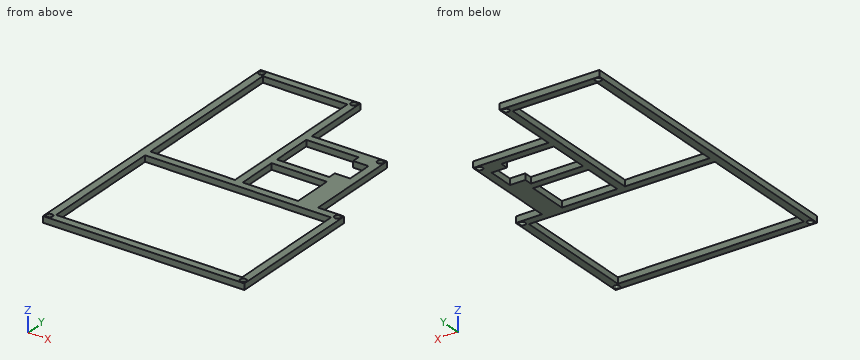
from build123d import *

# Parameters (mm, degrees)
F0_W     = 5
F0_H     = 5
F1_DEPTH = 4


with BuildPart() as f1:
    # F0 (on Top) → F1 (new body)
    with BuildSketch(Plane.XY):
        with BuildLine():
            Line((82.7990943193, -150.3260023594), (82.7990943193, -150.8260023594))
            Line((82.7990943193, -150.8260023594), (85.2990943193, -150.8260023594))
            Line((85.2990943193, -150.8260023594), (85.2990943193, -148.3260023594))
            Line((85.2990943193, -148.3260023594), (84.7990943193, -148.3260023594))
            ThreePointArc((84.7990943193, -148.3260023594), (84.2133078817, -149.7402159218), (82.7990943193, -150.3260023594))
        make_face()
        with BuildLine():
            Line((-45.2009056807, -148.3260023594), (-45.7009056807, -148.3260023594))
            Line((-45.7009056807, -148.3260023594), (-45.7009056807, -150.8260023594))
            Line((-45.7009056807, -150.8260023594), (-43.2009056807, -150.8260023594))
            Line((-43.2009056807, -150.8260023594), (-43.2009056807, -150.3260023594))
            ThreePointArc((-43.2009056807, -150.3260023594), (-44.615119243, -149.7402159218), (-45.2009056807, -148.3260023594))
        make_face()
        with BuildLine():
            Line((-43.2009056807, 49.1739976406), (-43.2009056807, 49.6739976406))
            Line((-43.2009056807, 49.6739976406), (-45.7009056807, 49.6739976406))
            Line((-45.7009056807, 49.6739976406), (-45.7009056807, 47.1739976406))
            Line((-45.7009056807, 47.1739976406), (-45.2009056807, 47.1739976406))
            ThreePointArc((-45.2009056807, 47.1739976406), (-44.615119243, 48.588211203), (-43.2009056807, 49.1739976406))
        make_face()
        with BuildLine():
            Line((85.2990943193, -61.3260023594), (85.2990943193, -58.8260023594))
            Line((85.2990943193, -58.8260023594), (82.7990943193, -58.8260023594))
            Line((82.7990943193, -58.8260023594), (82.7990943193, -59.3260023594))
            ThreePointArc((82.7990943193, -59.3260023594), (84.2133078817, -59.911788797), (84.7990943193, -61.3260023594))
            Line((84.7990943193, -61.3260023594), (85.2990943193, -61.3260023594))
        make_face()
        with BuildLine():
            Line((19.2990943193, 49.6739976406), (16.7990943193, 49.6739976406))
            Line((16.7990943193, 49.6739976406), (16.7990943193, 49.1739976406))
            ThreePointArc((16.7990943193, 49.1739976406), (18.2133078817, 48.588211203), (18.7990943193, 47.1739976406))
            Line((18.7990943193, 47.1739976406), (19.2990943193, 47.1739976406))
            Line((19.2990943193, 47.1739976406), (19.2990943193, 49.6739976406))
        make_face()
        with BuildLine():
            Line((85.2990943193, -63.8260023594), (85.2990943193, -61.3260023594))
            Line((85.2990943193, -61.3260023594), (84.7990943193, -61.3260023594))
            ThreePointArc((84.7990943193, -61.3260023594), (81.384880757, -62.7402159218), (82.7990943193, -59.3260023594))
            Line((82.7990943193, -59.3260023594), (82.7990943193, -58.8260023594))
            Line((82.7990943193, -58.8260023594), (80.2990943193, -58.8260023594))
            Line((80.2990943193, -58.8260023594), (80.2990943193, -63.8260023594))
            Line((80.2990943193, -63.8260023594), (85.2990943193, -63.8260023594))
        make_face()
        with BuildLine():
            Line((14.2990943193, 49.6739976406), (14.2990943193, 44.6739976406))
            Line((14.2990943193, 44.6739976406), (16.7990943193, 44.6739976406))
            Line((16.7990943193, 44.6739976406), (19.2990943193, 44.6739976406))
            Line((19.2990943193, 44.6739976406), (19.2990943193, 47.1739976406))
            Line((19.2990943193, 47.1739976406), (18.7990943193, 47.1739976406))
            ThreePointArc((18.7990943193, 47.1739976406), (15.384880757, 45.7597840782), (16.7990943193, 49.1739976406))
            Line((16.7990943193, 49.1739976406), (16.7990943193, 49.6739976406))
            Line((16.7990943193, 49.6739976406), (14.2990943193, 49.6739976406))
        make_face()
        with BuildLine():
            Line((-37.7009056807, -58.8260023594), (-40.7009056807, -58.8260023594))
            Line((-40.7009056807, -58.8260023594), (-40.7009056807, -52.8260023594))
            Line((-40.7009056807, -52.8260023594), (-40.7009056807, 28.4739976406))
            Line((-40.7009056807, 28.4739976406), (-40.7009056807, 44.6739976406))
            Line((-40.7009056807, 44.6739976406), (14.2990943193, 44.6739976406))
            Line((14.2990943193, 44.6739976406), (14.2990943193, 49.6739976406))
            Line((14.2990943193, 49.6739976406), (-43.2009056807, 49.6739976406))
            Line((-43.2009056807, 49.6739976406), (-43.2009056807, 49.1739976406))
            ThreePointArc((-43.2009056807, 49.1739976406), (-41.7866921183, 48.588211203), (-41.2009056807, 47.1739976406))
            ThreePointArc((-41.2009056807, 47.1739976406), (-43.2009056807, 45.1739976406), (-45.2009056807, 47.1739976406))
            Line((-45.2009056807, 47.1739976406), (-45.7009056807, 47.1739976406))
            Line((-45.7009056807, 47.1739976406), (-45.7009056807, -148.3260023594))
            Line((-45.7009056807, -148.3260023594), (-45.2009056807, -148.3260023594))
            ThreePointArc((-45.2009056807, -148.3260023594), (-43.2009056807, -146.3260023594), (-41.2009056807, -148.3260023594))
            ThreePointArc((-41.2009056807, -148.3260023594), (-41.7866921183, -149.7402159218), (-43.2009056807, -150.3260023594))
            Line((-43.2009056807, -150.3260023594), (-43.2009056807, -150.8260023594))
            Line((-43.2009056807, -150.8260023594), (82.7990943193, -150.8260023594))
            Line((82.7990943193, -150.8260023594), (82.7990943193, -150.3260023594))
            ThreePointArc((82.7990943193, -150.3260023594), (81.384880757, -146.911788797), (84.7990943193, -148.3260023594))
            Line((84.7990943193, -148.3260023594), (85.2990943193, -148.3260023594))
            Line((85.2990943193, -148.3260023594), (85.2990943193, -63.8260023594))
            Line((85.2990943193, -63.8260023594), (80.2990943193, -63.8260023594))
            Line((80.2990943193, -63.8260023594), (80.2990943193, -58.8260023594))
            Line((80.2990943193, -58.8260023594), (68.2990943193, -58.8260023594))
            Line((68.2990943193, -58.8260023594), (68.2990943193, -22.3260023594))
            Line((68.2990943193, -22.3260023594), (68.2990943193, -5.3260023594))
            Line((68.2990943193, -5.3260023594), (63.2990943193, -5.3260023594))
            Line((63.2990943193, -5.3260023594), (63.2990943193, -22.3260023594))
            Line((63.2990943193, -22.3260023594), (53.2990943193, -22.3260023594))
            Line((53.2990943193, -22.3260023594), (53.2990943193, -25.3760023594))
            Line((53.2990943193, -25.3760023594), (53.2990943193, -27.3260023594))
            Line((53.2990943193, -27.3260023594), (51.3490943193, -27.3260023594))
            Line((51.3490943193, -27.3260023594), (28.5490943193, -27.3260023594))
            Line((28.5490943193, -27.3260023594), (19.2990943193, -27.3260023594))
            Line((19.2990943193, -27.3260023594), (19.2990943193, -25.3760023594))
            Line((19.2990943193, -25.3760023594), (19.2990943193, -2.2760023594))
            Line((19.2990943193, -2.2760023594), (19.2990943193, -0.3260023594))
            Line((19.2990943193, -0.3260023594), (14.2990943193, -0.3260023594))
            Line((14.2990943193, -0.3260023594), (14.2990943193, -27.3260023594))
            Line((14.2990943193, -27.3260023594), (14.2990943193, -32.3260023594))
            Line((14.2990943193, -32.3260023594), (14.2990943193, -47.2260023594))
            Line((14.2990943193, -47.2260023594), (14.2990943193, -58.8260023594))
            Line((14.2990943193, -58.8260023594), (11.2990943193, -58.8260023594))
            Line((11.2990943193, -58.8260023594), (-37.7009056807, -58.8260023594))
        make_face()
        Polygon((76.8990943193, -63.8260023594), (80.2990943193, -63.8260023594), (80.2990943193, -67.2260023594), (80.2990943193, -142.4260023594), (80.2990943193, -145.8260023594), (76.8990943193, -145.8260023594), (-37.3009056807, -145.8260023594), (-40.7009056807, -145.8260023594), (-40.7009056807, -142.4260023594), (-40.7009056807, -67.2260023594), (-40.7009056807, -63.8260023594), (-37.3009056807, -63.8260023594), (14.2990943193, -63.8260023594), (19.2990943193, -63.8260023594), align=None, mode=Mode.SUBTRACT)
        Polygon((53.5990943193, -58.8260023594), (19.2990943193, -58.8260023594), (19.2990943193, -32.3260023594), (53.5990943193, -32.3260023594), (55.2990943193, -32.3260023594), (55.2990943193, -34.0260023594), (55.2990943193, -57.1260023594), (55.2990943193, -58.8260023594), align=None, mode=Mode.SUBTRACT)
        with Locations((16.7990943193, 2.1739976406)):
            Rectangle(F0_W, F0_H)
        Polygon((16.7990943193, 44.6739976406), (14.2990943193, 44.6739976406), (14.2990943193, 29.8739976406), (14.2990943193, 4.6739976406), (19.2990943193, 4.6739976406), (19.2990943193, 44.6739976406), align=None)
        with BuildLine():
            Line((65.7990943193, 4.6739976406), (19.2990943193, 4.6739976406))
            Line((19.2990943193, 4.6739976406), (19.2990943193, -0.3260023594))
            Line((19.2990943193, -0.3260023594), (28.5490943193, -0.3260023594))
            Line((28.5490943193, -0.3260023594), (51.3490943193, -0.3260023594))
            Line((51.3490943193, -0.3260023594), (53.2990943193, -0.3260023594))
            Line((53.2990943193, -0.3260023594), (53.2990943193, -2.2760023594))
            Line((53.2990943193, -2.2760023594), (53.2990943193, -5.3260023594))
            Line((53.2990943193, -5.3260023594), (63.2990943193, -5.3260023594))
            Line((63.2990943193, -5.3260023594), (68.2990943193, -5.3260023594))
            Line((68.2990943193, -5.3260023594), (68.2990943193, 2.1739976406))
            Line((68.2990943193, 2.1739976406), (67.7990943193, 2.1739976406))
            ThreePointArc((67.7990943193, 2.1739976406), (64.384880757, 0.7597840782), (65.7990943193, 4.1739976406))
            Line((65.7990943193, 4.1739976406), (65.7990943193, 4.6739976406))
        make_face()
        with BuildLine():
            Line((68.2990943193, 4.6739976406), (65.7990943193, 4.6739976406))
            Line((65.7990943193, 4.6739976406), (65.7990943193, 4.1739976406))
            ThreePointArc((65.7990943193, 4.1739976406), (67.2133078817, 3.588211203), (67.7990943193, 2.1739976406))
            Line((67.7990943193, 2.1739976406), (68.2990943193, 2.1739976406))
            Line((68.2990943193, 2.1739976406), (68.2990943193, 4.6739976406))
        make_face()
    extrude(amount=F1_DEPTH)


solid = f1.part
Geometry check sheet. Reference: the model listing, model coordinates, mm. Give positions to 0.01 mm unless a question says otherwise; leave off trailing zeros. Write each loop counter-clockwise with the first axis right and the second up, starting at its lowest first coordinate (ties: lowest second). Pieces come first, ordered by that corner, then holes.
1) Go/stop test with flat-tipped pins: pin 1 Ø2 at (x, z) = (38.5, 1) entering from +Y; pin 2 Ø1.2 at (y, z) = (17, 1.5) entering from +X; pin 3 Ø2 at (y, z) = (-48.5, 2) entering from +X; pin 4 Ø5 at (x, y) = (55.5, -21.5) entering from +Z. Record where each tip stops, or that it passes through.
Values follow:
pin 1: stops at y = 4.67
pin 2: stops at x = 19.3
pin 3: stops at x = 68.3
pin 4: stops at z = 4
2) Cross-section at C-C (x = -6). Record the boundary of the cut face in (y, z), plus the area to 3 significant figures.
Values follow:
outline: (-150.83, 0) - (-145.83, 0) - (-145.83, 4) - (-150.83, 4) - close; (-63.83, 0) - (-58.83, 0) - (-58.83, 4) - (-63.83, 4) - close; (44.67, 0) - (49.67, 0) - (49.67, 4) - (44.67, 4) - close
area: 60.0 mm2
3) Cross-section at B-B (y = -34.5). Record the boundary of the cut face in (x, z), plus the area to 3 significant figures.
Values follow:
outline: (-45.7, 0) - (-40.7, 0) - (-40.7, 4) - (-45.7, 4) - close; (14.3, 0) - (19.3, 0) - (19.3, 4) - (14.3, 4) - close; (55.3, 0) - (68.3, 0) - (68.3, 4) - (55.3, 4) - close
area: 92.0 mm2
4) Cross-section at A-A (x = 71.5). Record the boundary of the cut face in (y, z), plus the area to 3 significant figures.
Values follow:
outline: (-150.83, 0) - (-145.83, 0) - (-145.83, 4) - (-150.83, 4) - close; (-63.83, 0) - (-58.83, 0) - (-58.83, 4) - (-63.83, 4) - close
area: 40.0 mm2
5) Thickness scan on line 1 (Y direction, x = 5, z = 1.1); line 2 (Y direction, x = 20.5, z = 2.1); line 3 (X direction, y = -24, z = 0.6). Record the ranges inside material, lowest first.
Values follow:
line 1: y = -150.83 to -145.83, -63.83 to -58.83, 44.67 to 49.67
line 2: y = -150.83 to -145.83, -63.83 to -58.83, -32.33 to -27.33, -0.33 to 4.67
line 3: x = -45.7 to -40.7, 14.3 to 19.3, 53.3 to 68.3
6) Cross-section at D-D (y = -88.5). Record the boundary of the cut face in (x, z), plus the area to 3 significant figures.
Values follow:
outline: (-45.7, 0) - (-40.7, 0) - (-40.7, 4) - (-45.7, 4) - close; (80.3, 0) - (85.3, 0) - (85.3, 4) - (80.3, 4) - close
area: 40.0 mm2
